```python
from build123d import *

# Parameters (mm, degrees)
SKETCH_1_R          = 3.25
EXTRUDE_1_DEPTH     = 19.5
SKETCH_2_W          = 14
SKETCH_2_H          = 12
EXTRUDE_2_DEPTH     = 1
EXTRUDE_3_DEPTH     = 14
FILLET_1_R          = 2
SKETCH_5_W          = 19
SKETCH_5_H          = 19
EXTRUDE_4_DEPTH     = 1.5
SKETCH_6_R          = 1.5
CUT_EXTRUDE_1_DEPTH = 11.75
SKETCH_7_W          = 13
SKETCH_7_H          = 10
CUT_EXTRUDE_2_DEPTH = 2


with BuildPart() as part:
    # Sketch 1 → Extrude 1 (new body)
    with BuildSketch(Plane.XY):
        Circle(SKETCH_1_R)
    extrude(amount=EXTRUDE_1_DEPTH)



with BuildPart() as body_2:
    # Sketch 2 → Extrude 2 (new body)
    with BuildSketch(Plane(origin=(5, 0, 0), x_dir=(0, 0, -1), z_dir=(1, 0, 0))):
        with Locations((-9.75, 0)):
            Rectangle(SKETCH_2_W, SKETCH_2_H)
    extrude(amount=EXTRUDE_2_DEPTH)


with BuildPart() as part_1:
    add(part.part)

    add(body_2.part)  # Extrude 3 merges body 2
    # Sketch 3 → Extrude 3 (add)
    with BuildSketch(Plane(origin=(0, 0, 2.75), x_dir=(-1, 0, 0), z_dir=(0, 0, -1))):
        Polygon((0, 0), (-5, 4.5), (-5, -4.5), align=None)
    extrude(amount=-EXTRUDE_3_DEPTH)

    # Fillet 1
    fillet_1_edges = [part_1.edges().sort_by_distance(p)[0] for p in [
        (2.415705975, 2.174135378, 9.75),
        (2.415705975, -2.174135378, 9.75),
        (5, 4.5, 9.75),
        (5, -4.5, 9.75),
    ]]
    fillet(fillet_1_edges, radius=FILLET_1_R)

    # Sketch 5 → Extrude 4 (add)
    with BuildSketch(Plane(origin=(6, 0, 0), x_dir=(0, 0, -1), z_dir=(1, 0, 0))):
        with Locations((-9.75, 0)):
            Rectangle(SKETCH_5_W, SKETCH_5_H)
    extrude(amount=EXTRUDE_4_DEPTH)

    # Sketch 6 → Cut-Extrude 1 (cut, through all)
    with BuildSketch(Plane(origin=(7.5, 0, 0), x_dir=(0, 0, -1), z_dir=(1, 0, 0))):
        with Locations((-13, 0)):
            Circle(SKETCH_6_R)
        with Locations((-6.5, 0)):
            Circle(SKETCH_6_R)
    extrude(amount=-CUT_EXTRUDE_1_DEPTH, mode=Mode.SUBTRACT)

    # Sketch 7 → Cut-Extrude 2 (cut)
    with BuildSketch(Plane(origin=(7.5, 0, 0), x_dir=(0, 0, -1), z_dir=(1, 0, 0))):
        with Locations((-9.75, 0)):
            Rectangle(SKETCH_7_W, SKETCH_7_H)
    extrude(amount=-CUT_EXTRUDE_2_DEPTH, mode=Mode.SUBTRACT)


solid = part_1.part
```
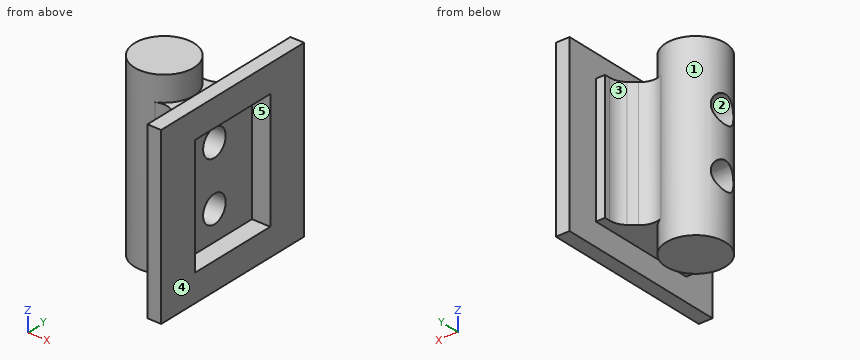
Geometry check sheet. Reference: the model listing, model coordinates, mm. Face numbers are marked on the shaded views. A direction names the side the tool comes from. Give positions to 0.01 mm unless a question says otherwise; leave off trailing zeros. Order: outer loops, then holes, each group sorted by start corner. A loop starts at its lowest first (then second) coordinate and runs counter-clockwise, first axis right, second up.
1. Thickness scan on L1, parallel to Z at x = 2, y = 0; L2, parallel to Z at x = 4.5, y = 0.5; L3, parallel to Z at x = 3.75, y = -2.5. Record the ranges inside material, lowest first.
2. Gauge pin test, flat ends, axial feed: pin 1 Ø2.5 at (y, z) = (0, 13) entering from -X; pin 2 Ø1 at (x, z) = (5, 4.5) entering from +Y; pin 3 Ø2 at (x, y) = (6, -0.5) entering from -Z; pin 4 Ø0.8 at (x, y) = (7, 2.5) entering from +Z. Record the tip position at first contact, or that the pin passes through.
3. Section check A-A, the plane x = 6.5. Enter the section's corners in (y, z).
4. Section check B-B, the plane z = 7. Enter the section's corners in (x, y).
5. Section check C-C, the plane x = 0. Enter the section's corners in (y, z).
6. Access from +Z, -Z, +X, -X, +Y, -Y to the whole of each face (thin tool, end or side, straight path). Record for the marked faces 4 and 5.
7. Section check D-D, the plane z = 9.5. Enter the section's corners in (x, y), and give its area (3 significant figures).
8. Release check for a two-part mould opening along X. For the marked faces 1, 2 and 3 record: pulls with the +X half, pulls with the -X half, needs draft (parallel to the pull), parting line crosses it, or undercut.
Values follow:
1. L1: z = 0 to 5, 8 to 11.5, 14.5 to 19.5
1. L2: z = 2.75 to 5.09, 7.91 to 11.59, 14.41 to 16.75
1. L3: z = 2.75 to 16.75
2. pin 1: passes through
2. pin 2: stops at y = 6
2. pin 3: stops at z = 0.25
2. pin 4: stops at z = 19.25
3. outline: (-9.5, 0.25) - (9.5, 0.25) - (9.5, 19.25) - (-9.5, 19.25) - close; hole (-5, 3.25) - (5, 3.25) - (5, 16.25) - (-5, 16.25) - close
4. outline: (-2.93, -1.41) arc R3.25 ccw to (1.41, -2.93) arc R2 cw to (3.61, -3.25) - (4.34, -3.9) arc R2 cw to (5, -5.39) - (5, -6) - (6, -6) - (6, -9.5) - (7.5, -9.5) - (7.5, -5) - (5.5, -5) - (5.5, -1.41) - close; (-2.93, 1.41) - (5.5, 1.41) - (5.5, 5) - (7.5, 5) - (7.5, 9.5) - (6, 9.5) - (6, 6) - (5, 6) - (5, 5.39) arc R2 cw to (4.34, 3.9) - (3.61, 3.25) arc R2 cw to (1.41, 2.93) arc R3.25 ccw to start
5. outline: (-3.25, 0) - (3.25, 0) - (3.25, 19.5) - (-3.25, 19.5) - close; hole circle Ø3 at (0, 6.5); hole circle Ø3 at (0, 13)
6. face 4: +Z, -Z, +X, +Y, -Y
6. face 5: +X
7. outline: (1.41, -2.93) arc R2 cw to (3.61, -3.25) - (4.34, -3.9) arc R2 cw to (5, -5.39) - (5, -6) - (6, -6) - (6, -9.5) - (7.5, -9.5) - (7.5, -5) - (5.5, -5) - (5.5, 5) - (7.5, 5) - (7.5, 9.5) - (6, 9.5) - (6, 6) - (5, 6) - (5, 5.39) arc R2 cw to (4.34, 3.9) - (3.61, 3.25) arc R2 cw to (1.41, 2.93) arc R3.25 ccw (long way) to start
7. area: 69.5 mm2
8. face 1: undercut
8. face 2: needs draft
8. face 3: pulls with the -X half
